Autodesk Inventor part; units mm, degrees
ref_plane "YZ Plane" through (0, 0, 0) normal (1, 0, 0) x (0, 1, 0)
ref_plane "XZ Plane" through (0, 0, 0) normal (0, 1, 0) x (-1, 0, 0)
ref_plane "XY Plane" through (0, 0, 0) normal (0, 0, 1) x (1, 0, 0)
sketch "スケッチ1" plane through (0, 0, 0) normal (0, 0, 1) x (1, 0, 0)
  line L0 (-16.7, 1.5) -> (16.7, 1.5) construction
  line L1 (16.7, 1.5) -> (16.7, -1.5) construction
  line L2 (16.7, -1.5) -> (-16.7, -1.5) construction
  line L3 (-16.7, -1.5) -> (-16.7, 1.5) construction
  line L4 (-16.7, 1.5) -> (16.7, -1.5) construction
  line L5 (16.7, 1.5) -> (-16.7, -1.5) construction
  line L6 (-16.7, -1.5) -> (-16.7, 1.5)
  line L7 (-16.7, 1.5) -> (16.7, 1.5)
  line L8 (16.7, 1.5) -> (16.7, -1.5)
  line L9 (16.7, -1.5) -> (18.7, -1.5)
  line L10 (18.7, -1.5) -> (18.7, 9.5)
  line L11 (18.7, 9.5) -> (-18.7, 9.5)
  line L12 (-18.7, 9.5) -> (-18.7, -1.5)
  line L13 (-18.7, -1.5) -> (-16.7, -1.5)
  circle A0 centre (-12.5, 5.5) radius 2.25
  line L14 (0, 9.5) -> (0, 0) construction
  circle A1 centre (12.5, 5.5) radius 2.25
  dimension "d0" = 3
  dimension "d1" = 33.4
  dimension "d2" = 8
  dimension "d3" = 2
  dimension "d4" = 4.5
  dimension "d5" = 4
  dimension "d6" = 6.2
extrude "押し出し1" add sketch "スケッチ1" along normal blind 1.8
sketch "スケッチ2" plane through (0, 0, 1.8) normal (0, 0, 1) x (1, 0, 0)
  line L0 (-18.7, -1.5) -> (-16.7, -1.5)
  line L1 (-16.7, -1.5) -> (-13.7, 1.5)
  line L2 (-13.7, 1.5) -> (13.7, 1.5)
  line L3 (13.7, 1.5) -> (16.7, -1.5)
  line L4 (16.7, -1.5) -> (18.7, -1.5)
  line L5 (18.7, -1.5) -> (18.7, 9.5)
  line L6 (18.7, 9.5) -> (-18.7, 9.5)
  line L7 (-18.7, 9.5) -> (-18.7, -1.5)
  line L8 (-16.7, 1.5) -> (16.7, 1.5)
  circle A0 centre (-12.5, 5.5) radius 2.25
  circle A1 centre (12.5, 5.5) radius 2.25
  point P0 (0, 0)
  dimension "d9" = 135
  dimension "d10" = 135
extrude "押し出し2" add sketch "スケッチ2" along normal blind 2.1
sketch "スケッチ3" plane through (0, 0, 0) normal (0, 0, -1) x (-1, 0, 0)
  circle A0 centre (-12.5, 5.5) radius 2.25
  circle A1 centre (12.5, 5.5) radius 2.25
  line L0 (18.7, -1.5) -> (16.7, -1.5)
  line L1 (16.7, -1.5) -> (13.7, 1.5)
  line L2 (13.7, 1.5) -> (-13.7, 1.5)
  line L3 (-13.7, 1.5) -> (-16.7, -1.5)
  line L4 (-16.7, -1.5) -> (-18.7, -1.5)
  line L5 (-18.7, -1.5) -> (-18.7, 9.5)
  line L6 (-18.7, 9.5) -> (18.7, 9.5)
  line L7 (18.7, 9.5) -> (18.7, -1.5)
  point P0 (0, 0)
extrude "押し出し3" add sketch "スケッチ3" along normal blind 2.1
fillet "フィレット1" radius 4 2 edges at (18.7, 9.5, 0.9) (-18.7, 9.5, 0.9)
equation "\"d5\" = 0.5 * d2"
equation "\"d10\" = d9"
properties part number "dcdcfixer" material "アルミニウム 6061"
Check sheet for the modelled part. Datum: model origin and axes. Units: mm. A direction names the side the tool comes from. Coordinates: 2 decimals unless noted, no trailing zeros. Order: outer loops, then holes, each group sorted by start corner. A loop starts at its lowest first (then second) coordinate and runs counter-clockwise, first axis right, second up. Notation, with made-up numbers: (-3.75, 45) -> (34.25, 45) arc R35 cw to (34.25, 81) -> close; hole circle Ø11 at (69.25, -6.5). An arc over 180 degrees is marked (long way). Write each question's results on one line, items separated by ' | '. Start each with the question number.
1) Set-up check for faces 1 (the face through (0, 9.5, 1)), 2 (the face through (16.7, 0, 1)), 3 (the face through (15.2, 0, -1)): record each of +Z, -Z, +X, -X, +Y, -Y from which the full face is reachable in a straight line by a thin tool's end or side.
2) Draft check along X on faces 4 (the face through (18.7, 2, 1)), 5 (the face through (0, 5, -2.1)), 6 (the face through (-16, 1, 0)). Enter one of: pulls with the +X half, pulls with the -X half, needs draft (parallel to the pull), parting line crosses it, or undercut.
3) Material ranges on line 1 along X through (y, z) = (5.5, -0.45); line 2 along Y through (x, z) = (-12.5, -0.8); line 3 along Y through (x, z) = (1, 1), recorded low to high.
4) Section check C-C (x = -12.5). Enter the section's corners in (y, z), and give its area (3 significant figures).
5) Section check A-A (y = -0.25). Enter the section's corners in (x, z).
6) Section check D-D (y = 6). Enter the section's corners in (x, z).
7) Depth check by flat-ended pin: pin 1 (3 mm diameter, centred on x = -7, z = 1, fed in from -Y); pin 2 (3 mm diameter, centred on y = 7.5, z = -1, fed in from -X). Enter the tip coordinate at first touch or a pass-through.
Checked values:
1) face 1: +Z, -Z, +X, -X, +Y | face 2: -Y | face 3: +Z, -Z, -Y
2) face 4: pulls with the +X half | face 5: needs draft | face 6: undercut
3) line 1: -18.7 to -14.75, -10.25 to 10.25, 14.75 to 18.7 | line 2: 1.5 to 3.25, 7.75 to 9.5 | line 3: 1.5 to 9.5
4) outline: (1.5, -2.1) -> (3.25, -2.1) -> (3.25, 3.9) -> (1.5, 3.9) -> close; (7.75, -2.1) -> (9.5, -2.1) -> (9.5, 3.9) -> (7.75, 3.9) -> close | area: 21.0 mm²
5) outline: (-18.7, -2.1) -> (-15.45, -2.1) -> (-15.45, 0) -> (-16.7, 0) -> (-16.7, 1.8) -> (-15.45, 1.8) -> (-15.45, 3.9) -> (-18.7, 3.9) -> close; (15.45, -2.1) -> (18.7, -2.1) -> (18.7, 3.9) -> (15.45, 3.9) -> (15.45, 1.8) -> (16.7, 1.8) -> (16.7, 0) -> (15.45, 0) -> close
6) outline: (-18.67, -2.1) -> (-14.69, -2.1) -> (-14.69, 3.9) -> (-18.67, 3.9) -> close; (-10.31, -2.1) -> (10.31, -2.1) -> (10.31, 3.9) -> (-10.31, 3.9) -> close; (14.69, -2.1) -> (18.67, -2.1) -> (18.67, 3.9) -> (14.69, 3.9) -> close
7) pin 1: y = 1.5 | pin 2: x = -18.67
